Part model, mm, in its own coordinate system. A direction names the side the tool comes from. Coordinates: 2 decimals unless noted, no trailing zeros. Loops run counter-clockwise (first coordinate to the right, second up) from the corner with the lowest first, then second, coordinate; pieces in that order, holes last. Notation, with made-up numbers: (-38.75, 73) -> (15.25, 73) arc R14 ccw to (15.25, 81) -> close; hole circle Ø7 at (-14, -33.75). An arc over 180 degrees is marked (long way). Use one line per item in the form item = value. Start each with the question number.
(1) Band-saw the part on A-A on x = 0. Give the cut face in (y, z).
(2) Pin check, flat tips, straight feed: P1, Ø6, axis at x = 0.5, y = 0, coming from the -Z side; P2, Ø4, axis at x = -1.5, z = 4.5, coming from the +Y side; P3, Ø4, axis at x = -6.5, z = 3, coming from the +Y side; P4, Ø1.8, axis at x = 1, z = 5.5, coming from the +Y side. Stop position of each tip, or through.
(3) Band-saw the part on B-B on y = 0.25. Give the cut face in (x, z), then the cut area to 3 significant figures.
(4) Mould opens along Y. For faces 1 (the flat face through (0, -13, 4)), 2 (the flat face through (7.24, -3.89, 1.48)), 3 (the flat face through (0, -4, 3)), 4 (the cylindrical face through (0, -2, 1)) say: +Y half, -Y half, draft (parallel to the pull), parting line (faces both ways), or undercut.
(5) Band-saw the part on C-C on z = 7.5. Give the cut face in (x, y), then the cut area to 3 significant figures.
(6) 3-axis set-ups, long thin cutter, end or side, ignore diameter. For faces 5 (the flat face through (0, -10, 6)), 6 (the cylindrical face through (0, 5, 1)): which of +Z, -Z, +X, -X, +Y, -Y reach the whole face in a straight line?
(7) Drill centre lines: L1, parallel to Y at x = 0, z = 2.3; L2, parallel to Z at x = 4, y = -4.5; L3, parallel to Y at x = 5.75, z = 7. Where is each one in solid material? Low to high. Write a range as [from, to].
(8) Band-saw the part on D-D on x = 5.5. Give the cut face in (y, z), then the cut area to 3 significant figures.
```python
from build123d import *

# Parameters (mm, degrees)
SKETCH_1_R      = 2
EXTRUDE_1_DEPTH = 3
SKETCH_2_W      = 20
SKETCH_2_H      = 3
EXTRUDE_2_DEPTH = 9


with BuildPart() as part:
    # 草图1 → 凸台-拉伸1 (new body)
    with BuildSketch(Plane.XY):
        with BuildLine():
            Line((0, -10), (-10, -10))
            Line((-10, -10), (-4.557189139, 2.057189139))
            ThreePointArc((-4.557189139, 2.057189139), (0, 5), (4.557189139, 2.057189139))
            Line((4.557189139, 2.057189139), (10, -10))
            Line((10, -10), (0, -10))
        make_face()
        Circle(SKETCH_1_R, mode=Mode.SUBTRACT)
    extrude(amount=EXTRUDE_1_DEPTH)

    # 草图2 → 凸台-拉伸2 (add)
    with BuildSketch(Plane(origin=(0, 0, 0), x_dir=(-1, 0, 0), z_dir=(0, 0, -1))):
        with Locations((0, -11.5)):
            Rectangle(SKETCH_2_W, SKETCH_2_H)
    extrude(amount=-EXTRUDE_2_DEPTH)


solid = part.part
```
A:
q1.outline = (-13, 0) -> (-2, 0) -> (-2, 3) -> (-10, 3) -> (-10, 9) -> (-13, 9) -> close; (2, 0) -> (5, 0) -> (5, 3) -> (2, 3) -> close
q2.P1 = 0
q2.P2 = 5
q2.P3 = 2.18
q2.P4 = -10
q3.outline = (-5.37, 0) -> (-1.98, 0) -> (-1.98, 3) -> (-5.37, 3) -> close; (1.98, 0) -> (5.37, 0) -> (5.37, 3) -> (1.98, 3) -> close
q3.area = 20.3 mm²
q4.face_1 = -Y half
q4.face_2 = +Y half
q4.face_3 = draft
q4.face_4 = undercut
q5.outline = (-10, -13) -> (10, -13) -> (10, -10) -> (-10, -10) -> close
q5.area = 60.0 mm²
q6.face_5 = +Z, +X, -X, +Y
q6.face_6 = +Z, -Z, +Y
q7.L1 = [-13, -2], [2, 5]
q7.L2 = [0, 3]
q7.L3 = [-13, -10]
q8.outline = (-13, 0) -> (-0.03, 0) -> (-0.03, 3) -> (-10, 3) -> (-10, 9) -> (-13, 9) -> close
q8.area = 56.9 mm²
